Verification items for the finished model (mm, model axes). A direction names the side the tool comes from. Round coordinates to 2 decimals unless told otherwise and drop trailing zeros. Order: outer loops, then holes, each group sorted by start corner. A loop starts at its lowest first (then second) coordinate and runs counter-clockwise, first axis right, second up. Notation, with made-up numbers: (89, 89.25) -> (143, 89.25) arc R21 cw to (143, 94.25) -> close; hole circle Ø2 at (25.5, 50). An arc over 180 degrees is marked (long way). Return JSON: item names as keys, results as strings. Group by question number.
Item 1: Depth check by flat-ended pin: pin 1 Ø4 at (x, y) = (-6.5, 3.5) entering from -Z; pin 2 Ø1.6 at (y, z) = (-1.5, -72) entering from +X; pin 3 Ø2.5 at (y, z) = (0, -67.5) entering from -X. Enter the tip coordinate at first touch or a pass-through.
Item 2: Sectioned sample at B-B on y = -1.5. Record the cut outline in (x, z), plus the area to 3 significant figures.
Item 3: Sectioned sample at D-D on z = -69. Record the cut outline in (x, y).
Item 4: Sectioned sample at A-A on x = 12. Record the cut outline in (y, z), plus the area to 3 significant figures.
Item 5: Access from +Z, -Z, +X, -X, +Y, -Y to the whole of each face (thin tool, end or side, straight path). Record for faces 1 (the flat face through (21, 0, -85)), 2 (the flat face through (9.647, 0, -72)), 3 (the flat face through (-1, -5, 1)), 4 (the flat face through (39, 0, -1)), 5 (the flat face through (21, -3.032, -72)).
Item 6: Scan lines: probe 1 along X at (y, z) = (-0.5, 15.5); probe 2 along Z at (x, y) = (-34.5, 3.75); probe 3 along Y at (x, z) = (23.5, -1.5). Record each from-to range of solid material in increasing order. Write a range as from..to.
Item 7: Draft check along Y on faces 6 (the flat face through (-39, 0, -1)), 7 (the flat face through (21, 2.217, -72)), 8 (the flat face through (32.81, 0, -72)). Enter one of: pulls with the +Y half, pulls with the -Y half, needs draft (parallel to the pull), parting line crosses it, or undercut.
Item 8: Sectioned sample at C-C on z = -22. Record the cut outline in (x, y), plus the area to 3 significant figures.
```python
from build123d import *

# Parameters (mm, degrees)
F0_W     = 80
F0_H     = 120
F1_DEPTH = 5
F2_T     = -1
F3_W     = 23.1627868488
F3_H     = 5.2490865346
F4_DEPTH = 25


with BuildPart() as f1:
    # F0 (on Front) → F1 (new body, symmetric)
    with BuildSketch(Plane.XZ):
        Rectangle(F0_W, F0_H)
    extrude(amount=F1_DEPTH, both=True)

    # F2 (hollow: no face is removed)
    offset(amount=F2_T, mode=Mode.SUBTRACT)

    # F3 (on face) → F4 (join)
    with BuildSketch(Plane(origin=(0, 0, -60), x_dir=(1, 0, 0), z_dir=(0, 0, -1))):
        with Locations((21.2281174026, 0.4071515286)):
            Rectangle(F3_W, F3_H)
    extrude(amount=F4_DEPTH)


solid = f1.part
```
Recorded:
{
 "1": {"pin 1": "z = -60", "pin 2": "x = 32.81", "pin 3": "x = 9.65"},
 "2": {"outline": "(-40, -60) -> (9.65, -60) -> (9.65, -85) -> (32.81, -85) -> (32.81, -60) -> (40, -60) -> (40, 60) -> (-40, 60) -> close; hole (-39, -59) -> (39, -59) -> (39, 59) -> (-39, 59) -> close", "area": "975 mm²"},
 "3": {"outline": "(9.65, -3.03) -> (32.81, -3.03) -> (32.81, 2.22) -> (9.65, 2.22) -> close"},
 "4": {"outline": "(-5, -60) -> (-3.03, -60) -> (-3.03, -85) -> (2.22, -85) -> (2.22, -60) -> (5, -60) -> (5, 60) -> (-5, 60) -> close; hole (-4, -59) -> (4, -59) -> (4, 59) -> (-4, 59) -> close", "area": "387 mm²"},
 "5": {"face 1": "-Z, +X, -X, +Y, -Y", "face 2": "-Z, -X, +Y, -Y", "face 3": "+Z, -Z, +X, -X, -Y", "face 4": "none", "face 5": "-Z, +X, -X, -Y"},
 "6": {"probe 1": "-40..-39, 39..40", "probe 2": "-60..-59, 59..60", "probe 3": "-5..-4, 4..5"},
 "7": {"face 6": "undercut", "face 7": "pulls with the +Y half", "face 8": "needs draft"},
 "8": {"outline": "(-40, -5) -> (40, -5) -> (40, 5) -> (-40, 5) -> close; hole (-39, -4) -> (39, -4) -> (39, 4) -> (-39, 4) -> close", "area": "176 mm²"}
}
